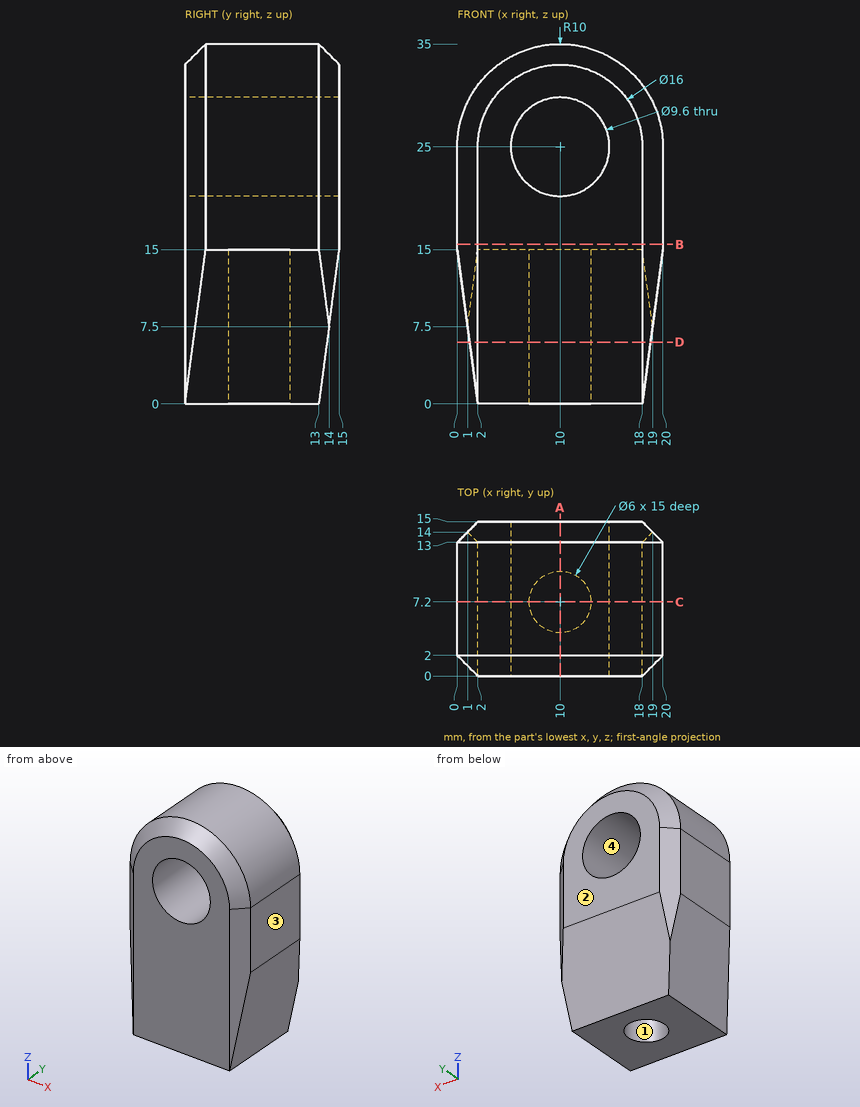
Geometry: see drawing. Coordinates: mm, zero at the bounding-box minimum. Coordinates: 2 decimals unless noted, no trailing zeros. Loops run counter-clockwise (first coordinate to the right, second up) from the corner with the lowest first, then second, coordinate; pieces in that order, holes last. Notation, with made-up numbers: (28.5, -8) - (69.5, -8) arc R22 ccw to (69.5, 10) - close; hole circle Ø5 at (-8, 36.25). An arc over 180 degrees is marked (long way). Answer in a Markdown table with one row per item.
(1) Cut plane B-B on z = 15.5. Output: boundary loops of the cut face in (x, y).
Model answer:
| item | result |
|---|---|
| outline | (0, 2) - (2, 0) - (18, 0) - (20, 2) - (20, 13) - (18, 15) - (2, 15) - (0, 13) - close |
(2) Cut plane C-C on y = 7.2. Output: boundary loops of the cut face in (x, z).
Model answer:
| item | result |
|---|---|
| outline | (0, 15) - (2, 0) - (7, 0) - (7, 15) - (13, 15) - (13, 0) - (18, 0) - (20, 15) - (20, 25) arc R10 ccw to (0, 25) - close; hole circle Ø9.6 at (10, 25) |
(3) Cut plane A-A on x = 10. Output: boundary loops of the cut face in (y, z), plus the area to 3 significant figures.
Model answer:
| item | result |
|---|---|
| outline | (0, 0) - (4.2, 0) - (4.2, 15) - (10.2, 15) - (10.2, 0) - (13, 0) - (15, 15) - (15, 20.2) - (0, 20.2) - close; (0, 29.8) - (15, 29.8) - (15, 33) - (13, 35) - (2, 35) - (0, 33) - close |
| area | 272 mm² |
(4) Pin query (flat end, axial travel): P1, Ø6, axis at x = 9, y = 6.5, coming from the -Z side; P2, Ø8, axis at x = 18, z = 8, coming from the +Y side; P3, Ø1.8, axis at x = 10, y = 6, coming from the -Z side; P4, Ø6, axis at x = 10, z = 25, coming from the -Y side. Return the tip coordinate at first contact, or that it passes through.
Model answer:
| item | result |
|---|---|
| P1 | stops at z = 0 |
| P2 | stops at y = 14.6 |
| P3 | stops at z = 15 |
| P4 | passes through |
(5) Material intervals for L1, parallel to Z at x = 10.5, y = 8.75; L2, parallel to X at y = 12.75, z = 28; L3, parallel to X at y = 6.5, z = 26, sorted ascending. Write a range as from..to.
Model answer:
| item | result |
|---|---|
| L1 | z = 15..20.23, 29.77..34.99 |
| L2 | x = 0.46..6.25, 13.75..19.54 |
| L3 | x = 0.05..5.31, 14.69..19.95 |
(6) Cut plane D-D on z = 6. Output: boundary loops of the cut face in (x, y), plus the area to 3 significant figures.
Model answer:
| item | result |
|---|---|
| outline | (1.2, 0.8) - (2, 0) - (18, 0) - (18.8, 0.8) - (18.8, 13.8) - (1.2, 13.8) - close; hole circle Ø6 at (10, 7.2) |
| area | 214 mm² |
(7) Mould query, pull axis X, two halves, no side actions, for the marked faces 1, 2, 3 and 4. Classes: pulls with the +X half, pulls with the -X half, needs draft (parallel to the pull), parting line crosses it, or undercut.
Model answer:
| item | result |
|---|---|
| face 1 | undercut |
| face 2 | needs draft |
| face 3 | pulls with the +X half |
| face 4 | undercut |
